```python
from build123d import *

# Parameters (mm, degrees)
SKETCH_1_W           = 136
SKETCH_1_H           = 40
EXTRUDE_1_DEPTH      = 2
SKETCH_3_R           = 1.6
CUT_EXTRUDE_3_DEPTH  = 71.908391605
CUT_EXTRUDE_5_DEPTH  = 71.908391605
SKETCH_7_W           = 136
SKETCH_7_H           = 8
CUT_EXTRUDE_6_DEPTH  = 71.908391605
CUT_EXTRUDE_7_DEPTH  = 71.908391605
CUT_EXTRUDE_START    = -2
CUT_EXTRUDE_8_DEPTH  = 2
FILLET_2_R           = 1
FILLET_3_R           = 1
SKETCH_11_W          = 26
SKETCH_11_H          = 3
CUT_EXTRUDE_9_DEPTH  = 71.908391605
FILLET_4_R           = 0.5
SKETCH_13_W          = 6
SKETCH_13_H          = 28
SKETCH_13_R          = 1.6
EXTRUDE_2_DEPTH      = 2
SKETCH_14_R          = 1.6
CUT_EXTRUDE_10_DEPTH = 10
FILLET_5_R           = 1
FILLET_6_R           = 1


# Read off the part's stored shape, not the designer's step: 切除-拉伸8
with BuildPart() as part:
    # 草图1 → 凸台-拉伸1 (new body)
    with BuildSketch(Plane.XY):
        Rectangle(SKETCH_1_W, SKETCH_1_H)
    extrude(amount=EXTRUDE_1_DEPTH)

    # 草图3 → 切除-拉伸3 (cut, through all)
    with BuildSketch(Plane.XY.offset(2)):
        with Locations((65, -5)):
            Circle(SKETCH_3_R)
        with Locations((65, 15)):
            Circle(SKETCH_3_R)
        with Locations((-65, 15)):
            Circle(SKETCH_3_R)
        with Locations((-65, -5)):
            Circle(SKETCH_3_R)
    extrude(amount=-CUT_EXTRUDE_3_DEPTH, mode=Mode.SUBTRACT)

    # 草图6 → 切除-拉伸5 (cut, through all)
    with BuildSketch(Plane.XY.offset(2)):
        with BuildLine():
            Line((26.513057993, -6.191225838), (29.496623679, -5.877640448))
            ThreePointArc((29.496623679, -5.877640448), (27.848048141, -4.5426503), (26.513057993, -6.191225838))
        make_face()
        Polygon((29.716133451, -7.966136428), (29.496623679, -5.877640448), (26.513057993, -6.191225838), (26.732567765, -8.279721818), align=None)
        with BuildLine():
            ThreePointArc((26.732567765, -8.279721818), (28.381143303, -9.614711966), (29.716133451, -7.966136428))
            Line((29.716133451, -7.966136428), (26.732567765, -8.279721818))
        make_face()
        Polygon((38.66683051, -7.025380259), (38.447320737, -4.936884279), (29.496623679, -5.877640448), (29.716133451, -7.966136428), align=None)
        Polygon((41.650396196, -6.711794869), (41.430886423, -4.623298889), (38.447320737, -4.936884279), (38.66683051, -7.025380259), align=None)
        with BuildLine():
            Line((38.447320737, -4.936884279), (41.430886423, -4.623298889))
            ThreePointArc((41.430886423, -4.623298889), (39.782310885, -3.288308741), (38.447320737, -4.936884279))
        make_face()
        with BuildLine():
            ThreePointArc((38.66683051, -7.025380259), (40.315406048, -8.360370407), (41.650396196, -6.711794869))
            Line((41.650396196, -6.711794869), (38.66683051, -7.025380259))
        make_face()
    cut_extrude_5 = extrude(amount=-CUT_EXTRUDE_5_DEPTH, mode=Mode.SUBTRACT)

    # 镜向1: 切除-拉伸5 across plane
    add(cut_extrude_5.mirror(Plane(origin=(0, 0, 0), x_dir=(0, 0, 1), z_dir=(1, 0, 0))), mode=Mode.SUBTRACT)

    # 草图7 → 切除-拉伸6 (cut, through all)
    with BuildSketch(Plane.XY.offset(2)):
        with Locations((0, -16)):
            Rectangle(SKETCH_7_W, SKETCH_7_H)
    extrude(amount=-CUT_EXTRUDE_6_DEPTH, mode=Mode.SUBTRACT)

    # 草图8 → 切除-拉伸7 (cut, through all)
    with BuildSketch(Plane.XY.offset(2)):
        Polygon((-68, -7), (-68, -12), (-20.428177729, -12), align=None)
        Polygon((20.428177729, -12), (68, -7), (68, -12), align=None)
    extrude(amount=-CUT_EXTRUDE_7_DEPTH, mode=Mode.SUBTRACT)

    # 切除-拉伸8 outline → 切除-拉伸8 (cut)
    with BuildSketch(Plane.XY.offset(2).offset(CUT_EXTRUDE_START)):
        Polygon((18.456507715, 10.75175987), (2.313148778, -3), (18.456507715, -3), align=None)
        Polygon((-18.456507715, 10.75175987), (-18.456507715, -3), (-2.313148778, -3), align=None)
        Polygon((-62, 12.092619933), (-62, 1.418949104), (-46.311418135, -0.229987295), align=None)
        Polygon((-21.456507715, 11.312594625), (-41.066399544, -0.781260963), (-21.456507715, -2.842343647), align=None)
        Polygon((-59.571610636, 14), (-43.404423487, 1.301471928), (-22.814069976, 14), align=None)
        Polygon((43.404423487, 1.301471928), (59.571610636, 14), (22.814069976, 14), align=None)
        Polygon((-14.121622282, 11), (-1.5, 0.24824013), (-1.5, 11), align=None)
        Polygon((1.5, 0.24824013), (14.121622282, 11), (1.5, 11), align=None)
        Polygon((41.066399544, -0.781260963), (21.456507715, 11.312594625), (21.456507715, -2.842343647), align=None)
        Polygon((62, 12.092619933), (46.311418135, -0.229987295), (62, 1.418949104), align=None)
    extrude(amount=CUT_EXTRUDE_8_DEPTH, mode=Mode.SUBTRACT)

    # 圆角2
    fillet_2_edges = [part.edges().sort_by_distance(p)[0] for p in [
        (-68, -7, 1),
        (-20.428177729, -12, 1),
        (20.428177729, -12, 1),
        (68, -7, 1),
        (-68, 20, 1),
        (68, 20, 1),
    ]]
    fillet(fillet_2_edges, radius=FILLET_2_R)

    # 圆角3
    fillet_3_edges = [part.edges().sort_by_distance(p)[0] for p in [
        (14.121622282, 11, 1),
        (1.5, 0.24824013, 1),
        (1.5, 11, 1),
        (46.311418135, -0.229987295, 1),
        (62, 12.092619933, 1),
        (62, 1.418949104, 1),
        (21.456507715, 11.312594625, 1),
        (41.066399544, -0.781260963, 1),
        (21.456507715, -2.842343647, 1),
        (43.404423487, 1.301471928, 1),
        (22.814069976, 14, 1),
        (59.571610636, 14, 1),
        (-18.456507715, -3, 1),
        (-18.456507715, 10.75175987, 1),
        (-2.313148778, -3, 1),
        (-1.5, 11, 1),
        (-1.5, 0.24824013, 1),
        (-14.121622282, 11, 1),
        (-43.404423487, 1.301471928, 1),
        (-59.571610636, 14, 1),
        (-22.814069976, 14, 1),
        (-21.456507715, -2.842343647, 1),
        (-41.066399544, -0.781260963, 1),
        (-21.456507715, 11.312594625, 1),
        (-46.311418135, -0.229987295, 1),
        (-62, 1.418949104, 1),
        (-62, 12.092619933, 1),
        (18.456507715, -3, 1),
        (2.313148778, -3, 1),
        (18.456507715, 10.75175987, 1),
        (29.496623679, -5.877640448, 1),
        (38.447320737, -4.936884279, 1),
        (38.66683051, -7.025380259, 1),
        (29.716133451, -7.966136428, 1),
        (-29.496623679, -5.877640448, 1),
        (-29.716133451, -7.966136428, 1),
        (-38.66683051, -7.025380259, 1),
        (-38.447320737, -4.936884279, 1),
    ]]
    fillet(fillet_3_edges, radius=FILLET_3_R)

    # 草图11 → 切除-拉伸9 (cut, through all)
    with BuildSketch(Plane(origin=(0, 0, 0), x_dir=(-1, 0, 0), z_dir=(0, 0, -1))):
        with BuildLine():
            Line((-6.4, 16.25), (-6.4, 14.75))
            ThreePointArc((-6.4, 14.75), (-8, 13.15), (-9.6, 14.75))
            Line((-9.6, 14.75), (-9.6, 16.25))
            ThreePointArc((-9.6, 16.25), (-8, 17.85), (-6.4, 16.25))
        make_face()
        with BuildLine():
            Line((9.6, 16.25), (9.6, 14.75))
            ThreePointArc((9.6, 14.75), (8, 13.15), (6.4, 14.75))
            Line((6.4, 14.75), (6.4, 16.25))
            ThreePointArc((6.4, 16.25), (8, 17.85), (9.6, 16.25))
        make_face()
        with Locations((0, 20)):
            Rectangle(SKETCH_11_W, SKETCH_11_H)
    extrude(amount=-CUT_EXTRUDE_9_DEPTH, mode=Mode.SUBTRACT)

    # 圆角4
    fillet_4_edges = [part.edges().sort_by_distance(p)[0] for p in [
        (13, 20, 1),
        (-13, 20, 1),
        (13, 18.5, 1),
        (-13, 18.5, 1),
    ]]
    fillet(fillet_4_edges, radius=FILLET_4_R)

    # 草图13 → 凸台-拉伸2 (add)
    # profile 1 of 2: a face of its own
    with BuildSketch(Plane(origin=(0, 0, 0), x_dir=(-1, 0, 0), z_dir=(0, 0, -1))):
        with Locations((-65, -4)):
            Rectangle(SKETCH_13_W, SKETCH_13_H)
        with Locations((-65, -15)):
            Circle(SKETCH_13_R, mode=Mode.SUBTRACT)
    # profile 2 of 2: a face of its own
    with BuildSketch(Plane(origin=(0, 0, 0), x_dir=(-1, 0, 0), z_dir=(0, 0, -1))):
        with Locations((65, -4)):
            Rectangle(SKETCH_13_W, SKETCH_13_H)
        with Locations((65, -15)):
            Circle(SKETCH_13_R, mode=Mode.SUBTRACT)
    extrude(amount=-EXTRUDE_2_DEPTH)

    # 草图14 → 切除-拉伸10 (cut)
    with BuildSketch(Plane(origin=(0, 0, 0), x_dir=(-1, 0, 0), z_dir=(0, 0, -1))):
        with Locations((-65, 5)):
            Circle(SKETCH_14_R)
        with Locations((-65, -5)):
            Circle(SKETCH_14_R)
    cut_extrude_10 = extrude(amount=-CUT_EXTRUDE_10_DEPTH, mode=Mode.SUBTRACT)

    # 圆角5
    fillet_5_edges = [part.edges().sort_by_distance(p)[0] for p in [
        (68, -18, 1),
        (62, -7.630625412, 1),
        (62, -18, 1),
    ]]
    fillet(fillet_5_edges, radius=FILLET_5_R)

    # 镜向4: 切除-拉伸10 across plane
    add(cut_extrude_10.mirror(Plane(origin=(0, 0, 0), x_dir=(0, 0, 1), z_dir=(1, 0, 0))), mode=Mode.SUBTRACT)

    # 圆角6
    fillet_6_edges = [part.edges().sort_by_distance(p)[0] for p in [
        (-62, -18, 1),
        (-62, -7.630625412, 1),
        (-68, -18, 1),
    ]]
    fillet(fillet_6_edges, radius=FILLET_6_R)


solid = part.part
```
Could you check a few things on this model? Use its own coordinates, in mm. A direction names the side the tool comes from. Round coordinates to 2 decimals unless told otherwise and drop trailing zeros. Loops run counter-clockwise (first coordinate to the right, second up) from the corner with the lowest first, then second, coordinate; pieces in that order, holes last. Notation, with made-up numbers: (74, 56.25) - (131, 56.25) arc R31 ccw to (131, 93.25) - close; hole circle Ø9 at (85, 77.5). An arc over 180 degrees is marked (long way). Use CSV: the item, a comma, the result in double quotes.
Item 1: I need wall thicknesses on L1, parallel to Y at x = 65, z = 1.35; L2, parallel to X at y = -13, z = 1.4; L3, parallel to Y at x = 35.5, z = 0.25. Which ranges of each line are inside material? Lowest first, please. Write a range as [from, to].
Here are the results:
L1,"y = [-18, -16.6], [-13.4, -6.6], [-3.4, 3.4], [6.6, 13.4], [16.6, 20]"
L2,"x = [-68, -62], [62, 68]"
L3,"y = [-10.42, -7.36], [-5.25, -1.37], [2.65, 6.18], [14, 20]"
Item 2: If we section it at C-C on x = 8: List the corners of the cut face in (y, z) for me, then the cut area to 3 significant figures.
Here are the results:
outline,"(-12, 0) - (-3, 0) - (-3, 2) - (-12, 2) - close; (1.84, 0) - (5.79, 0) - (5.79, 2) - (1.84, 2) - close; (11, 0) - (13.15, 0) - (13.15, 2) - (11, 2) - close; (17.85, 0) - (18.5, 0) - (18.5, 2) - (17.85, 2) - close"
area,"31.5 mm²"
Item 3: If we section it at A-A on x = 65: List the corners of the cut face in (y, z) for me, then the cut area to 3 significant figures.
Here are the results:
outline,"(-18, 0) - (-16.6, 0) - (-16.6, 2) - (-18, 2) - close; (-13.4, 0) - (-6.6, 0) - (-6.6, 2) - (-13.4, 2) - close; (-3.4, 0) - (3.4, 0) - (3.4, 2) - (-3.4, 2) - close; (6.6, 0) - (13.4, 0) - (13.4, 2) - (6.6, 2) - close; (16.6, 0) - (20, 0) - (20, 2) - (16.6, 2) - close"
area,"50.4 mm²"
Item 4: For faces 1 (the flat face through (-40.4, -9.9, 1)), 2 (the flat face through (10.681, 4.128, 0.986)), which set-ups out of +Z, -Z, +X, -X, +Y, -Y let a thin tool reach every point of the face, with its end or its side?
Here are the results:
face 1,"+Z, -Z, -Y"
face 2,"+Z, -Z"
Item 5: If we section it at D-D on y = 5: Count the separate pieces of the cut face and the enclosed holes in it, then the cut area to 3 significant figures.
Here are the results:
separate pieces,"13"
enclosed holes,"0"
area,"90.0 mm²"
Item 6: If we mould it in two halves opening along X, with no side actions, what happens to faces 3 (the flat face through (1, 5, 2)), 4 (the flat face through (34.194, 6.982, 0.986))? For each: pulls with the +X half, pulls with the -X half, needs draft (parallel to the pull), parting line crosses it, or undercut.
Here are the results:
face 3,"needs draft"
face 4,"undercut"
Item 7: If we section it at B-B on x = 47: List the corners of the cut face in (y, z) for me.
Here are the results:
outline,"(-9.21, 0) - (4.13, 0) - (4.13, 2) - (-9.21, 2) - close; (14, 0) - (20, 0) - (20, 2) - (14, 2) - close"
Item 8: Will these pins go through, and if not, where does the flat tip stop? pin 1 (1.9 mm diameter, centred on x = 65, y = 15, fed in from -Z); pin 2 (1 mm diameter, centred on x = 36.5, z = 1, fed in from -Y); pin 3 (1 mm diameter, centred on x = -9.5, z = 1.5, fed in from +Y).
Here are the results:
pin 1,"passes through"
pin 2,"stops at y = -10.36"
pin 3,"stops at y = 18.5"
